Source: CAD feature listing. Evaluate the final solid. Frame: model axes, mm. A direction names the side the tool comes from. Give positions to 0.01 mm unless a question says otherwise; leave off trailing zeros. Write each loop counter-clockwise with the first axis right and the second up, starting at its lowest first coordinate (ties: lowest second). Pieces come first, ordered by that corner, then holes. Notation, with made-up numbers: M 81,14.5 L 107,14.5 A24 ccw 107,36.5 Z; hole C -11.5,61 d8. An arc over 180 degrees is marked long. Answer as a JSON object with one key per item and string values. Group by question number.
```python
from build123d import *

# Parameters (mm, degrees)
SKETCH1_W           = 35
SKETCH1_H           = 35
BOSS_EXTRUDE1_DEPTH = 1
SKETCH2_W           = 12
SKETCH2_H           = 12
BOSS_EXTRUDE2_DEPTH = 22
SKETCH3_R           = 11.5
SKETCH3_R_2         = 10.25
BOSS_EXTRUDE3_DEPTH = 10


with BuildPart() as part:
    # Sketch1 → Boss-Extrude1 (new body)
    with BuildSketch(Plane(origin=(0, 0, 0), x_dir=(1, 0, 0), z_dir=(0, 1, 0))):
        with Locations((17.5, 17.5)):
            Rectangle(SKETCH1_W, SKETCH1_H)
    extrude(amount=BOSS_EXTRUDE1_DEPTH)

    # Sketch2 → Boss-Extrude2 (add)
    with BuildSketch(Plane(origin=(0, 1, 0), x_dir=(1, 0, 0), z_dir=(0, 1, 0))):
        with Locations((6, 29)):
            Rectangle(SKETCH2_W, SKETCH2_H)
    extrude(amount=BOSS_EXTRUDE2_DEPTH)

    # Sketch3 → Boss-Extrude3 (add)
    with BuildSketch(Plane.XZ):
        with Locations(Location((17.5, -17.5, 0), (0, 0, 270))):
            Circle(SKETCH3_R)
        with Locations(Location((17.5, -17.5, 0), (0, 0, 270))):
            Circle(SKETCH3_R_2, mode=Mode.SUBTRACT)
    extrude(amount=BOSS_EXTRUDE3_DEPTH)


solid = part.part
```
(1) Ray query, L1, parallel to X at y = -3, z = -17; L2, parallel to Y at x = 28, z = -32; L3, parallel to Y at x = 10.5, z = -28. Return the intervals inside material, ascending. Write a range as [from, to].
(2) Pull-direction query (Z, two-part tool) for faces 1 (the cylindrical face through (20.579, -4.93, -27.277)), 2 (the flat face through (6, 12, -23)), 3 (the flat face through (17, 1, -18)), 4 (the flat face through (17, 0, -18)); classes: pulls with the +Z half, pulls with the -Z half, needs draft (parallel to the pull), parting line crosses it, or undercut.
(3) Section C-C, the plane y = -6. Return loops of the section in (x, z), plus the area to 3 significant figures.
(4) Section D-D, the plane y = 18. Return loops of the section in (x, z).
(5) Section B-B, the plane x = 17.5. Return loops of the section in (y, z), plus the area to 3 significant figures.
(6) Section A-A, the plane z = -17.5. Return loops of the section in (x, y), plus the area to 3 significant figures.
(7) Access query for faces 5 (the cylindrical face through (20.95, -4.93, -28.47)), 6 (the flat face through (12, 12, -29)), 7 (the flat face through (0, 11, -28)). Directions: +Z, -Z, +X, -X, +Y, -Y. A direction counts if a zero-diameter tool reaches every point of the face in a straight line with its end or side. Return the directions, or none.
(8) Contact query for flat-ended pins moving along their axis: pin 1 Ø4 at (x, z) = (27.5, -3.5) entering from +Y; pin 2 Ø13 at (x, y) = (9, 15.5) entering from +Z; pin 3 Ø6 at (x, z) = (18, -18.5) entering from -Y. Output: stop coordinate, or through.
Reported:
{
 "1": {"L1": "x = [6.01, 7.26], [27.74, 28.99]", "L2": "y = [0, 1]", "L3": "y = [0, 23]"},
 "2": {"face 1": "undercut", "face 2": "pulls with the +Z half", "face 3": "needs draft", "face 4": "undercut"},
 "3": {"outline": "C 17.5,-17.5 d23; hole C 17.5,-17.5 d20.5", "area": "85.4 mm2"},
 "4": {"outline": "M 0,-35 L 12,-35 L 12,-23 L 0,-23 Z"},
 "5": {"outline": "M -10,-29 L 0,-29 L 0,-35 L 1,-35 L 1,0 L 0,0 L 0,-6 L -10,-6 L -10,-7.25 L 0,-7.25 L 0,-27.75 L -10,-27.75 Z", "area": "60.0 mm2"},
 "6": {"outline": "M 0,0 L 6,0 L 6,-10 L 7.25,-10 L 7.25,0 L 27.75,0 L 27.75,-10 L 29,-10 L 29,0 L 35,0 L 35,1 L 0,1 Z", "area": "60.0 mm2"},
 "7": {"face 5": "-Y", "face 6": "+Z, -Z, +X, +Y", "face 7": "+Z, -Z, -X, +Y, -Y"},
 "8": {"pin 1": "stops at y = 1", "pin 2": "stops at z = -23", "pin 3": "stops at y = 0"}
}
